Here's how the part is built. I have some questions about the finished solid (model axes, mm). A direction names the side the tool comes from. Coordinates: 2 decimals unless noted, no trailing zeros. Write each loop counter-clockwise with the first axis right and the second up, starting at its lowest first coordinate (ties: lowest second). Pieces come first, ordered by that corner, then holes. Notation, with made-up numbers: (-16.75, -0.5) -> (-0.75, -0.5) arc R29 ccw to (-0.75, 29.5) -> close; hole circle Ø3 at (42, 52). An arc over 180 degrees is marked (long way). Put each result on its own line as item: value. Start each with the question number.
Item 1: On a 3-axis mill with a long thin cutter (end or side, diameter ignored), from which of +Z, -Z, +X, -X, +Y, -Y can I reach the whole of each face in a straight line? I mean faces 4 (the face through (115.07, 15.92, 11.03)), 5 (the face through (28.246, 12.243, 5.499)), 6 (the face through (59, 14, 25.4)). Say none if no direction works.
Item 2: I want a section at A-A, the plane x = 108. List the corners of the cut face in (y, z) for me, then the cut area to 3 significant figures.
Item 3: I want a section at B-B, the plane z = 11.5. State how many separate pieces and enclosed holes the cut face has, then the cut area to 3 significant figures.
Item 4: For pin 1 (4 mm diameter, centred on x = 10.12, z = 12.7, fed in from -Y); pin 2 (8 mm diameter, centred on x = 109.77, z = 12.7, fed in from +Y), each with a flat end and sliding along its axis, tell me the tip position at first contact or that it passes through.
Item 5: If we mould it in two halves opening along Y, with no side actions, what happens to faces 1 (the face through (8.56, 6.26, 15.7)), 2 (the face through (59.105, 4.765, 22.798)), 3 (the face through (94.286, 12.243, 5.499))? For each: released by +Y, released by -Y, zero draft, split by the parting line, or undercut.
Item 6: I need wall thicknesses on line 1 (X direction, y = 2.5, z = 12.7); line 2 (X direction, y = 13.75, z = 5.75); line 3 (Y direction, x = 91.5, z = 9). Which ranges of each line are inside material? Lowest first, please. Write a range as [from, to].
from build123d import *

# Parameters (mm, degrees)
BOSS_EXTRUDE1_DEPTH                              = 119.888
CBORE_FOR_1_4_SOCKET_HEAD_CAP_SCREW1_D           = 6.7564
CBORE_FOR_1_4_SOCKET_HEAD_CAP_SCREW1_CBORE_D     = 11.1125
CBORE_FOR_1_4_SOCKET_HEAD_CAP_SCREW1_CBORE_DEPTH = 6.35
F_5_16_18_TAPPED_HOLE1_D                         = 6.5278
SKETCH6_R                                        = 6.35
CUT_EXTRUDE1_DEPTH                               = 125.150820709


with BuildPart() as part:
    # Sketch1 → Boss-Extrude1 (new body)
    with BuildSketch(Plane(origin=(0, 0, 0), x_dir=(0, 0, -1), z_dir=(1, 0, 0))):
        Polygon((0, 0), (0, 19.05), (-25.4, 19.05), (-25.4, 9.398), (-20.121342373, 0), align=None)
    extrude(amount=BOSS_EXTRUDE1_DEPTH)

    # CBORE for 1/4 Socket Head Cap Screw1 (through all)
    with Locations(Plane(origin=(0, 19.05, 0), x_dir=(1, 0, 0), z_dir=(0, 1, 0))):
        with Locations((10.11555, -12.7), (109.77245, -12.7)):
            CounterBoreHole(CBORE_FOR_1_4_SOCKET_HEAD_CAP_SCREW1_D / 2, CBORE_FOR_1_4_SOCKET_HEAD_CAP_SCREW1_CBORE_D / 2, CBORE_FOR_1_4_SOCKET_HEAD_CAP_SCREW1_CBORE_DEPTH)

    # 5/16-18 Tapped Hole1 (through all)
    with Locations(Plane(origin=(0, 4.568628166, -8.133879962), x_dir=(1, 0, 0), z_dir=(0, 0.48971726622701756, -0.8718812987781861))):
        with Locations((92.964, -16.609338742), (26.924, -16.609338742)):
            Hole(F_5_16_18_TAPPED_HOLE1_D / 2)

    # Sketch6 → Cut-Extrude1 (cut, through all)
    with BuildSketch(Plane(origin=(0, 0.588206226, -1.047228766), x_dir=(1, 0, 0), z_dir=(0, -0.48971726622701756, 0.8718812987781861))):
        with Locations((26.924, 16.609338742)):
            Circle(SKETCH6_R)
        with Locations((92.964, 16.609338742)):
            Circle(SKETCH6_R)
    extrude(amount=-CUT_EXTRUDE1_DEPTH, mode=Mode.SUBTRACT)


solid = part.part
Calculated:
1. face 4: +Y
1. face 5: none
1. face 6: +Z, +X, -X, +Y, -Y
2. outline: (0, 0) -> (19.05, 0) -> (19.05, 7.43) -> (12.7, 7.43) -> (12.7, 9.82) -> (0, 9.82) -> close; (0, 15.58) -> (12.7, 15.58) -> (12.7, 17.97) -> (19.05, 17.97) -> (19.05, 25.4) -> (9.4, 25.4) -> (0, 20.12) -> close
2. area: 319 mm2
3. separate pieces: 3
3. enclosed holes: 2
3. area: 1,910 mm2
4. pin 1: passes through
4. pin 2: stops at y = 12.7
5. face 1: zero draft
5. face 2: released by -Y
5. face 3: undercut
6. line 1: x = [0, 6.74], [13.49, 106.39], [113.15, 119.89]
6. line 2: x = [0, 20.84], [33.01, 86.88], [99.05, 119.89]
6. line 3: y = [0, 10.65], [17.34, 18.48]
